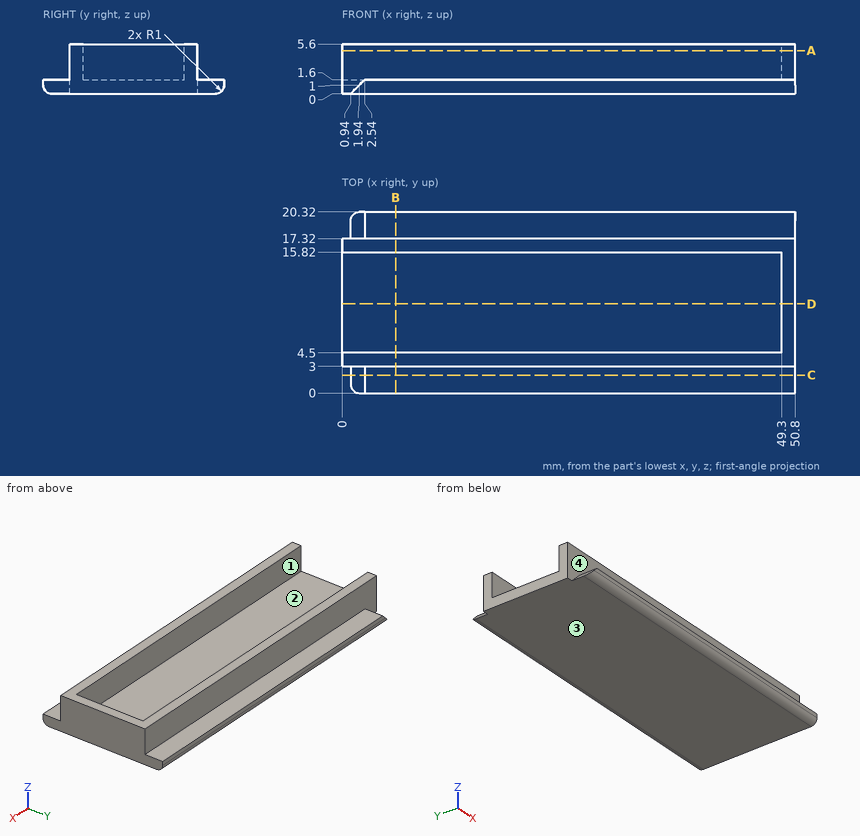
The figure shows three views and two pictorial views of one solid part (mm, origin at its lowest corner). Answer the questions. Give positions to 0.01 mm unless a question says otherwise; leave off trailing zeros. Write each loop counter-clockwise with the first axis right and the second up, starting at its lowest first coordinate (ties: lowest second). Pieces come first, ordered by that corner, then holes. Notation, with made-up numbers: M -14,13.25 L 37,13.25 A25 ccw 37,43.25 Z; hole C 73.5,40.25 d2. An arc over 180 degrees is marked long. Write each question's results on one line, items separated by ' | '.
Q1. Section D-D, the plane y = 10 is taken. Write down the section's boundary in (x, z), then the cut area to 3 significant figures.
Output values:
outline: M 0,0 L 50.8,0 L 50.8,5.6 L 49.3,5.6 L 49.3,1.6 L 0,1.6 Z | area: 87.3 mm2
Q2. Consider L1, parallel to Y at x = 6.5, z = 3.1; L2, parallel to Z at x = 35.5, y = 9; L3, parallel to X at y = 15.25, z = 3. Determine where each line is inside the solid, lowest interval first. Write a range as from..to.
Output values:
L1: 3..4.5, 15.82..17.32 | L2: 0..1.6 | L3: 49.3..50.8
Q3. Section C-C, the plane y = 2 is taken. Write down the section's boundary in (x, z).
Output values:
outline: M 0.94,0 L 50.8,0 L 50.8,1.6 L 2.54,1.6 Z
Q4. Flat-ended cylindrical pins translate along their axes: P1, Ø1, axis at y = 7.5, z = 5, coming from the -X side; P2, Ø1.7, axis at x = 30.5, z = 3.5, coming from the -Y side; P3, Ø1.2, axis at x = 23.5, z = 3.5, coming from the +Y side. Find the tip coordinate at first contact, or state that the pin passes through.
Output values:
P1: x = 49.3 | P2: y = 3 | P3: y = 17.32
Q5. Section B-B, the plane x = 6 is taken. Write down the section's boundary in (y, z), then the cut area to 3 significant figures.
Output values:
outline: M 0,1 A1 ccw 1,0 L 19.32,0 A1 ccw 20.32,1 L 20.32,1.6 L 17.32,1.6 L 17.32,5.6 L 15.82,5.6 L 15.82,1.6 L 4.5,1.6 L 4.5,5.6 L 3,5.6 L 3,1.6 L 0,1.6 Z | area: 44.1 mm2
Q6. For a pull along Y with two mould halves and no side action, classify the marked faces 1, 2, 3 and 4 as released by +Y, released by -Y, zero draft, split by the parting line, or undercut.
Output values:
face 1: undercut | face 2: undercut | face 3: zero draft | face 4: released by -Y
Q7. Section A-A, the plane z = 4.85 is taken. Write down the section's boundary in (x, y), then the cut area to 3 significant figures.
Output values:
outline: M 0,3 L 50.8,3 L 50.8,17.32 L 0,17.32 L 0,15.82 L 49.3,15.82 L 49.3,4.5 L 0,4.5 Z | area: 169 mm2
